For this review, take the finished solid that the model builds, in its own axes (mm). Face numbers are marked on the shaded views. A direction names the side the tool comes from. Coordinates: 2 decimals unless noted, no trailing zeros. Order: outer loops, then holes, each group sorted by start corner. A loop starts at its lowest first (then second) coordinate and runs counter-clockwise, first axis right, second up. Notation, with made-up numbers: (-18.5, 6) -> (-0.5, 6) arc R26 ccw to (-0.5, 32) -> close; hole circle Ø4 at (-11.5, 61.25). An arc over 180 degrees is marked (long way). Write item = value, one per line. Start each with the question number.
1) Consider section A-A on y = 0. Give the boundary of the cut face in (x, z), and give its area (4 significant figures).
2) Consider section D-D on y = -18.75. State how many separate pieces and enclosed holes the cut face has, and give its area (3 significant figures).
3) Consider section B-B on x = 0. Give the boundary of the cut face in (y, z).
4) Wall thickness on probe 1 along Y at (x, z) = (0, 1.15); probe 2 along X at (y, z) = (-18.75, 1.8); probe 3 along Z at (x, y) = (11, 28): over which ranges is each line inside the solid? List them lowest first. Write a range as [from, to].
5) Consider section C-C on z = 12.5. Give the boundary of the cut face in (x, y) (3 decimals).
6) Machinability: for the marked faces 4 and 5, which of the approach directions +Z, -Z, +X, -X, +Y, -Y give a long, thin tool a straight path to every point of the face, cutting with its end or side? Answer none if there is none.
7) Insertion check: pin 1 Ø5 at (y, z) = (20, 16.5) entering from +X; pin 2 Ø6 at (x, z) = (-4, 13.5) entering from -Y; pin 3 Ø1.5 at (x, z) = (-23, 15.5) entering from +Y. Each pin has a flat end and moves straight along its axis. Give the tip position at first contact, or say it passes through.
8) Draft analysis for pull direction X (two halves, no side actions). For the marked faces 1, 2 and 3, state which applies: +X half, -X half, draft (parallel to the pull), parting line (faces both ways), or undercut.
from build123d import *

# Parameters (mm, degrees)
SKETCH1_R           = 25
SKETCH1_R_2         = 5
BOSS_EXTRUDE1_DEPTH = 20
CUT_EXTRUDE2_DEPTH  = 65.097993278
CUT_EXTRUDE5_DEPTH  = 65.09799338
SKETCH17_W          = 27.497524216
SKETCH17_H          = 10
CUT_EXTRUDE7_DEPTH  = 69.272212154
CIRPATTERN1_COUNT   = 3


with BuildPart() as part:
    # Sketch1 → Boss-Extrude1 (new body)
    with BuildSketch(Plane.XY):
        with BuildLine():
            Line((-7.72740661, 39.570552361), (-9.859096528, 31.614977283))
            ThreePointArc((-9.859096528, 31.614977283), (-11.344452128, 28.681851078), (-13.884081425, 26.593839192))
            ThreePointArc((-13.884081425, 26.593839192), (-25.980762114, 15), (-29.972981037, -1.272952374))
            ThreePointArc((-29.972981037, -1.272952374), (-30.511437725, -4.516341804), (-32.308921731, -7.26926059))
            Line((-32.308921731, -7.26926059), (-38.132806891, -13.093145751))
            ThreePointArc((-38.132806891, -13.093145751), (-39.404155872, -22.75), (-30.405400281, -26.47740661))
            Line((-30.405400281, -26.47740661), (-22.449825203, -24.345716693))
            ThreePointArc((-22.449825203, -24.345716693), (-19.166985597, -24.165509274), (-16.088899612, -25.320886818))
            ThreePointArc((-16.088899612, -25.320886818), (0, -30), (16.088899612, -25.320886818))
            ThreePointArc((16.088899612, -25.320886818), (19.166985597, -24.165509274), (22.449825203, -24.345716693))
            Line((22.449825203, -24.345716693), (30.405400281, -26.47740661))
            ThreePointArc((30.405400281, -26.47740661), (39.404155872, -22.75), (38.132806891, -13.093145751))
            Line((38.132806891, -13.093145751), (32.308921731, -7.26926059))
            ThreePointArc((32.308921731, -7.26926059), (30.511437725, -4.516341804), (29.972981037, -1.272952374))
            ThreePointArc((29.972981037, -1.272952374), (25.980762114, 15), (13.884081425, 26.593839192))
            ThreePointArc((13.884081425, 26.593839192), (11.344452128, 28.681851078), (9.859096528, 31.614977283))
            Line((9.859096528, 31.614977283), (7.72740661, 39.570552361))
            ThreePointArc((7.72740661, 39.570552361), (0, 45.5), (-7.72740661, 39.570552361))
        make_face()
        Circle(SKETCH1_R, mode=Mode.SUBTRACT)
        with Locations((0, 37.5)):
            Circle(SKETCH1_R_2, mode=Mode.SUBTRACT)
        with Locations((32.475952642, -18.75)):
            Circle(SKETCH1_R_2, mode=Mode.SUBTRACT)
        with Locations((-32.475952642, -18.75)):
            Circle(SKETCH1_R_2, mode=Mode.SUBTRACT)
    extrude(amount=BOSS_EXTRUDE1_DEPTH)

    # Sketch14 → Cut-Extrude2 (cut, through all)
    with BuildSketch(Plane(origin=(0, 0, 0), x_dir=(-0.7071067811865461, 0.707106781186549, 0), z_dir=(-0.707106781186549, -0.7071067811865461, 0))):
        with BuildLine():
            Line((19.111501151, -15), (5, -15))
            ThreePointArc((5, -15), (0, -10), (5, -5))
            Line((5, -5), (19.111501151, -5))
            ThreePointArc((19.111501151, -5), (24.111501151, -10), (19.111501151, -15))
        make_face()
    cut_extrude2 = extrude(amount=-CUT_EXTRUDE2_DEPTH, mode=Mode.SUBTRACT)

    # Sketch15 → Cut-Extrude5 (cut, through all)
    with BuildSketch(Plane(origin=(0, 0, 0), x_dir=(0.7071067811865489, 0.7071067811865462, 0), z_dir=(-0.7071067811865462, 0.7071067811865489, 0))):
        with BuildLine():
            Line((17.551379006, -15), (5, -15))
            ThreePointArc((5, -15), (0, -10), (5, -5))
            Line((5, -5), (17.551379006, -5))
            ThreePointArc((17.551379006, -5), (22.551379006, -10), (17.551379006, -15))
        make_face()
    cut_extrude5 = extrude(amount=CUT_EXTRUDE5_DEPTH, mode=Mode.SUBTRACT)

    # Sketch17 → Cut-Extrude7 (cut, through all)
    with BuildSketch(Plane(origin=(0, 21.213203436, 0), x_dir=(-1, 0, 0), z_dir=(0, -1, 0))):
        with Locations((-1.299865662, -10)):
            Rectangle(SKETCH17_W, SKETCH17_H)
    cut_extrude7 = extrude(amount=-CUT_EXTRUDE7_DEPTH, mode=Mode.SUBTRACT)

    # CirPattern1: Cut-Extrude2, Cut-Extrude5, Cut-Extrude7 ×3 about axis
    cirpattern1_axis = Axis((0, 0, 0), (0, 0, 1))
    add([cut_extrude2.rotate(cirpattern1_axis, i * 360 / CIRPATTERN1_COUNT) for i in range(1, CIRPATTERN1_COUNT)], mode=Mode.SUBTRACT)
    add([cut_extrude5.rotate(cirpattern1_axis, i * 360 / CIRPATTERN1_COUNT) for i in range(1, CIRPATTERN1_COUNT)], mode=Mode.SUBTRACT)
    add([cut_extrude7.rotate(cirpattern1_axis, i * 360 / CIRPATTERN1_COUNT) for i in range(1, CIRPATTERN1_COUNT)], mode=Mode.SUBTRACT)


solid = part.part
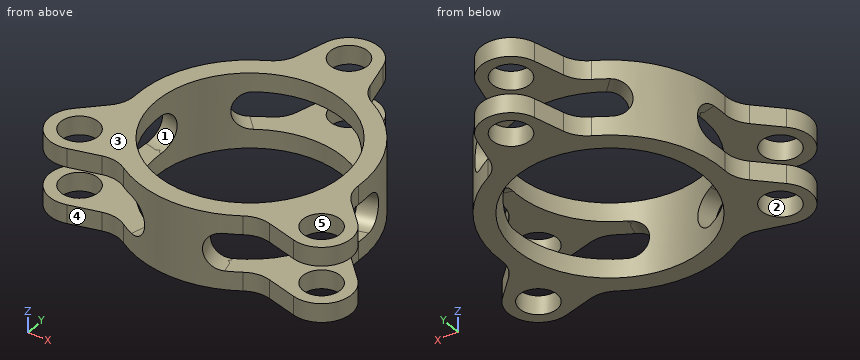
Answer sheet:
q1.outline = (-30, 0) -> (-25, 0) -> (-25, 5) -> (-30, 5) -> close; (-30, 15) -> (-25, 15) -> (-25, 20) -> (-30, 20) -> close; (25, 0) -> (30, 0) -> (30, 5) -> (25, 5) -> close; (25, 15) -> (30, 15) -> (30, 20) -> (25, 20) -> close
q1.area = 100.0 mm2
q2.separate_pieces = 8
q2.enclosed_holes = 0
q2.area = 279 mm2
q3.outline = (-30, 0) -> (-25, 0) -> (-25, 20) -> (-30, 20) -> close; (25, 0) -> (32.5, 0) -> (32.5, 5) -> (25, 5) -> close; (25, 15) -> (32.5, 15) -> (32.5, 20) -> (25, 20) -> close; (42.5, 0) -> (45.5, 0) -> (45.5, 5) -> (42.5, 5) -> close; (42.5, 15) -> (45.5, 15) -> (45.5, 20) -> (42.5, 20) -> close
q4.probe_1 = [-30, -25], [25, 32.5], [42.5, 45.5]
q4.probe_2 = [-40.48, -37.48], [-27.48, -16.54], [16.54, 27.48], [37.48, 40.48]
q4.probe_3 = [0, 5], [15, 20]
q5.outline = (-29.144, 7.116) -> (-24.313, 5.821) arc R25 cw to (-17.198, 18.145) -> (-20.734, 21.682) arc R30 ccw to start; (-8.41, -28.797) arc R30 ccw to (8.41, -28.797) -> (7.115, -23.966) arc R25 cw to (-7.115, -23.966) -> close; (17.198, 18.145) arc R25 cw to (24.313, 5.821) -> (29.144, 7.116) arc R30 ccw to (20.734, 21.682) -> close
q6.face_4 = +Z, -Z, -Y
q6.face_5 = +Z, -Z
q7.pin_1 = 24.37
q7.pin_2 = -29.98
q7.pin_3 = 20.12
q8.face_1 = -X half
q8.face_2 = undercut
q8.face_3 = draft
